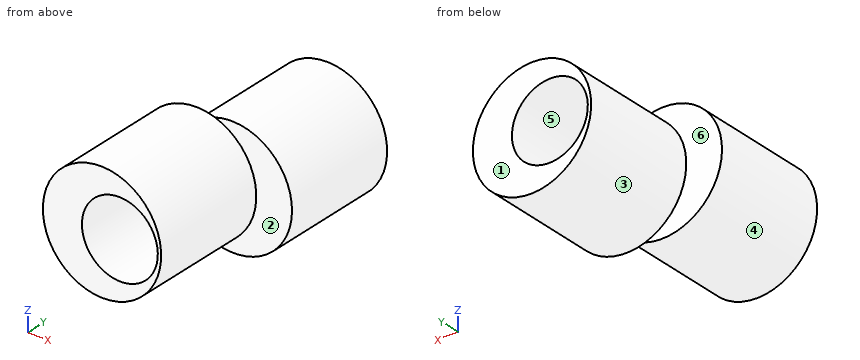
from build123d import *

# Parameters (mm, degrees)
SKETCH1_R               = 3.975
BOSS_EXTRUDE1_DEPTH     = 8
SKETCH1_3_R             = 3.975
BOSS_EXTRUDE2_DEPTH     = 8
CUT_EXTRUDE1_DEPTH      = 8
CUT_EXTRUDE1_DEPTH_BACK = 8
SKETCH1_5_R             = 2.55


with BuildPart() as part:
    # Sketch1 → Boss-Extrude1 (new body)
    with BuildSketch(Plane(origin=(0, 0, 0), x_dir=(1, 0, 0), z_dir=(0, 1, 0))):
        with Locations(Location((0, 0, 0), (0, 0, 270))):
            Circle(SKETCH1_R)
    extrude(amount=BOSS_EXTRUDE1_DEPTH)

    # Sketch1<3> → Boss-Extrude2 (add)
    with BuildSketch(Plane(origin=(0, 0, 0), x_dir=(1, 0, 0), z_dir=(0, 1, 0))):
        with Locations(Location((-2.4, 0, 0), (0, 0, 270))):
            Circle(SKETCH1_3_R)
    extrude(amount=-BOSS_EXTRUDE2_DEPTH)

    # Sketch1<5> → Cut-Extrude1 (cut, two sides: drawn at the far end of the back side and taken through both)
    with BuildSketch(Plane(origin=(0, 0, 0), x_dir=(1, 0, 0), z_dir=(0, 1, 0)).offset(-CUT_EXTRUDE1_DEPTH_BACK)):
        with Locations(Location((-1.2, 0, 0), (0, 0, 270))):
            Circle(SKETCH1_5_R)
    extrude(amount=CUT_EXTRUDE1_DEPTH + CUT_EXTRUDE1_DEPTH_BACK, mode=Mode.SUBTRACT)


solid = part.part
The model under review builds one solid part; all positions refer to its coordinate system, in mm. Face numbers are marked on the shaded views. A direction names the side the tool comes from. Round coordinates to 2 decimals unless told otherwise and drop trailing zeros. Order: outer loops, then holes, each group sorted by start corner. A loop starts at its lowest first (then second) coordinate and runs counter-clockwise, first axis right, second up. Notation, with made-up numbers: (-18.75, 67) -> (34.25, 67) arc R5 cw to (34.25, 76) -> close; hole circle Ø1 at (-32.5, 75.5). An arc over 180 degrees is marked (long way). Use CSV: the item, a comma, the result in double quotes. Start each with the question number.
(1) Consider section A-A on z = 0. Write out the cut boundary in (x, y) (3 decimals), and give its area (3 significant figures).
(2) Consider section D-D on x = -5.25. Write out the cut boundary in (y, z).
(3) Insertion check: pin 1 (1.5 mm diameter, centred on y = 1, z = -2.5, fed in from -X); pin 2 (1.5 mm diameter, centred on x = 0, y = -5, fed in from +Z); pin 3 (3 mm diameter, centred on y = -2.5, z = -2.5, fed in from -X). Each pin has a flat end and moves straight along its axis. Give the tip position at first contact, or say it passes through.
(4) Consider section C-C on y = 2. Write out the cut boundary in (x, z) (3 decimals).
(5) Tool access review of the marked faces 1, 2 and 3: name each direction out of +Z, -Z, +X, -X, +Y, -Y from which nothing blocks a thin tool from reaching the whole face with its end or side.
(6) Mouldability with a two-part tool opening along X and no side actions: class the marked faces 4, 5 and 6 as pulls with the +X half, pulls with the -X half, needs draft (parallel to the pull), parting line crosses it, or undercut.
(7) Wall thickness on probe 1 along X at (y, z) = (4.25, 0) (3 decimals); probe 2 along Y at (x, z) = (-5.5, 0.5); probe 3 along X at (y, z) = (4.25, 1): over which ranges is each line inside the solid? List them lowest first. Write a range as from..to.
(8) Consider section B-B on x = -2.4. Write out the cut boundary in (y, z) (3 decimals), and give its area (3 significant figures).
Responses:
1,outline,"(-6.375, -8) -> (-3.75, -8) -> (-3.75, 8) -> (-3.975, 8) -> (-3.975, 0) -> (-6.375, 0) -> close; (1.35, -8) -> (1.575, -8) -> (1.575, 0) -> (3.975, 0) -> (3.975, 8) -> (1.35, 8) -> close"
1,area,"45.6 mm²"
2,outline,"(-8, -2.77) -> (0, -2.77) -> (0, 2.77) -> (-8, 2.77) -> close"
3,pin 1,"x = -3.57"
3,pin 2,"z = 3.62"
3,pin 3,"x = -6.25"
4,outline,"circle Ø7.95 at (0, 0); hole circle Ø5.1 at (-1.2, 0)"
5,face 1,"+Z, -Z, +X, -X, +Y"
5,face 2,"+X, -Y"
5,face 3,"+Y"
6,face 4,"parting line crosses it"
6,face 5,"undercut"
6,face 6,"needs draft"
7,probe 1,"-3.975..-3.75, 1.35..3.975"
7,probe 2,"-8..0"
7,probe 3,"-3.85..-3.55, 1.15..3.85"
8,outline,"(-8, -3.975) -> (0, -3.975) -> (0, -3.169) -> (8, -3.169) -> (8, -2.25) -> (-8, -2.25) -> close; (-8, 2.25) -> (8, 2.25) -> (8, 3.169) -> (0, 3.169) -> (0, 3.975) -> (-8, 3.975) -> close"
8,area,"42.3 mm²"
